Autodesk Inventor part; units mm, degrees
ref_plane "Start Plane" through (0, 0, 25) normal (0, 0, 1) x (1, 0, 0)
ref_plane "End Plane" through (0, 0, 2285) normal (0, 0, 1) x (1, 0, 0)
ref_plane "Work Plane4" through (-235, -21, 25) normal (0, 0, -1) x (-1, 0, 0)
ref_plane "Start Plane" through (0, 0, 25) normal (0, 0, 1) x (1, 0, 0)
ref_plane "End Plane" through (0, 0, 2285) normal (0, 0, 1) x (1, 0, 0)
sketch "Sketch" plane through (0, 0, 0) normal (0, 0, 1) x (1, 0, 0)
  line L0 (-25, -21) -> (-25, 21)
  line L1 (-21, 25) -> (21, 25)
  line L2 (25, 21) -> (25, -21)
  line L3 (21, -25) -> (-21, -25)
  arc A0 (-25, -21) -> (-21, -25) centre (-21, -21) ccw
  arc A1 (25, 21) -> (21, 25) centre (21, 21) ccw
  arc A2 (-21, 25) -> (-25, 21) centre (-21, 21) ccw
  arc A3 (21, -25) -> (25, -21) centre (21, -21) ccw
  arc A4 (-21, 23) -> (-23, 21) centre (-21, 21) ccw
  line L4 (-21, 23) -> (21, 23)
  arc A5 (23, 21) -> (21, 23) centre (21, 21) ccw
  line L5 (23, 21) -> (23, -21)
  arc A6 (21, -23) -> (23, -21) centre (21, -21) ccw
  line L6 (21, -23) -> (-21, -23)
  arc A7 (-23, -21) -> (-21, -23) centre (-21, -21) ccw
  line L7 (-23, -21) -> (-23, 21)
  line L8 (0, 36.1598) -> (0, -36.1598) construction
  line L9 (-36.1598, 0) -> (36.1598, 0) construction
  dimension "d7" = 4
  dimension "d9" = 50
  dimension "d11" = 50
  dimension "d12" = 2
  dimension "d15" = 25
  dimension "d16" = 25
extrude "Body" add sketch "Sketch" along normal up to surface (2260 mm away) from surface at 25
sketch "Sketch3" plane through (0, 0, 0) normal (0, 0, 1) x (1, 0, 0)
  line L0 (0, 0) -> (10, 0)
ref_plane "Work Plane3" through (0, 0, 0) normal (0, -1, 0) x (1, 0, 0)
sketch "Sketch4" plane through (0, 0, 0) normal (0, -1, 0) x (1, 0, 0)
  line L0 (-2, 25) -> (12, 25)
  line L1 (-2, 2285) -> (12, 2285)
  dimension "d18" = 2260
ref_plane "Work Plane4" through (-235, -21, 25) normal (0, 0, -1) x (-1, 0, 0)
split "Split1" plane through (-235, -21, 25) removes the side toward (0, 0, -1)
ref_plane "Work Plane5" through (-235, 21, 2285) normal (0, 0, 1) x (1, 0, 0)
split "Split2" plane through (-235, 21, 2285) removes the side toward (0, 0, 1)
equation "\"d7\" = G_IR"
equation "\"d9\" = G_W"
equation "\"d11\" = G_H"
equation "\"d12\" = G_T"
equation "\"d15\" = 0.5 * d9"
equation "\"d16\" = 0.5 * d11"
equation "\"d3\" = G_L"
equation "\"G_W\" = 50"
equation "\"G_H\" = 50"
equation "\"G_T\" = 2"
equation "\"G_IR\" = 4"
equation "\"G_L\" = d18"
equation "\"G_OFFSET_START\" = -25"
equation "\"G_OFFSET_END\" = -25"
equation "\"d13\" = -G_OFFSET_START"
equation "\"d14\" = G_OFFSET_END + B_L"
properties part number "ISO 10799-2 - 50x50x2 - 2260"
Check sheet for the modelled part. Datum: model origin and axes. Units: mm. A direction names the side the tool comes from. Give positions to 0.01 mm unless a question says otherwise; leave off trailing zeros. Loops run counter-clockwise (first coordinate to the right, second up) from the corner with the lowest first, then second, coordinate; pieces in that order, holes last. Notation, with made-up numbers: M -31.5,86 L 8.5,86 A30 cw 8.5,122 Z; hole C 74.25,57.5 d11. An arc over 180 degrees is marked long. Answer as a JSON object with one key per item and string values. Group by question number.
Q1. Cross-section at A-A on x = 11.5. Record the cut outline in (y, z).
Q2. Cross-section at C-C on z = 1756. Record the cut outline in (x, y), then the cut area to 3 significant figures.
Q3. Release check for a two-part mould opening along X. For faces 3 (the flat face through (-23, 0, 1139)), 4 (the flat face through (0, 25, 1139)), 5 (the flat face through (-25, 0, 1139)) record: released by +X, released by -X, zero draft, split by the parting line, or undercut.
Q4. Access from +Z, -Z, +X, -X, +Y, -Y to the whole of each face (thin tool, end or side, straight path). Record for faces 1 (the flat face through (0, 24, 25)), 2 (the flat face through (23, 0, 1139)).
Q5. Material ranges on line 1 along Y through (x, z) = (5.5, 284); line 2 along X through (y, z) = (-21.5, 156.5), recorded low to high. Write a range as [from, to].
Evaluation:
{
 "1": {"outline": "M -25,25 L -23,25 L -23,2285 L -25,2285 Z; M 23,25 L 25,25 L 25,2285 L 23,2285 Z"},
 "2": {"outline": "M -25,-21 A4 ccw -21,-25 L 21,-25 A4 ccw 25,-21 L 25,21 A4 ccw 21,25 L -21,25 A4 ccw -25,21 Z; hole M -23,-21 A2 ccw -21,-23 L 21,-23 A2 ccw 23,-21 L 23,21 A2 ccw 21,23 L -21,23 A2 ccw -23,21 Z", "area": "374 mm2"},
 "3": {"face 3": "undercut", "face 4": "zero draft", "face 5": "released by -X"},
 "4": {"face 1": "-Z, +X, -X, +Y, -Y", "face 2": "+Z, -Z"},
 "5": {"line 1": "y = [-25, -23], [23, 25]", "line 2": "x = [-24.97, -22.94], [22.94, 24.97]"}
}
